Verification items for the finished model (mm, model axes). Face numbers are marked on the shaded views. A direction names the side the tool comes from. Round coordinates to 2 decimals unless told otherwise and drop trailing zeros. Write each loop counter-clockwise with the first axis right and the second up, starting at its lowest first coordinate (ties: lowest second). Pieces come first, ordered by that corner, then holes. Notation, with made-up numbers: M 2,58 L 31,58 A23 cw 31,87 Z; hole C 60.25,87 d3. An arc over 180 degrees is marked long. One line per item, written item: value. Start each with the question number.
Item 1: Gauge pin test, flat ends, axial feed: pin 1 (3.5 mm diameter, centred on x = 1, y = -17.5, fed in from +Z); pin 2 (2 mm diameter, centred on y = -5, z = 11, fed in from +X); pin 3 (1.6 mm diameter, centred on y = -19, z = -3.5, fed in from -X); pin 4 (13 mm diameter, centred on x = 19.64, z = -15, fed in from +Y). Record the tip position at first contact, or that the pin passes through.
Item 2: Tool access check on the marked faces 1 and 2. Record the directions out of +Z, -Z, +X, -X, +Y, -Y that give a thin tool (end or side, any length) a straight path to the whole face; none if there is none.
Item 3: Section check B-B, the plane y = -14. Record the cut outline in (x, z).
Item 4: Section check D-D, the plane x = 23. Record the cut outline in (y, z), then the cut area to 3 significant figures.
Item 5: Section check A-A, the plane x = 1. Record the cut outline in (y, z), then the cut area to 3 significant figures.
Item 6: Thickness scan on probe 1 along X at (y, z) = (-19, 15); probe 2 along X at (y, z) = (-1, 5.5); probe 3 along Y at (x, z) = (8.5, 0). Record the ranges inside material, lowest first. Write a range as from..to.
Item 7: Section check C-C, the plane z = 0. Record the cut outline in (x, y).
from build123d import *

# Parameters (mm, degrees)
SKETCH1_R           = 2.5
SKETCH1_W           = 35
SKETCH1_H           = 8
BOSS_EXTRUDE1_DEPTH = 1.5
BOSS_EXTRUDE2_DEPTH = 30
FILLET1_R           = 5
SKETCH2_R           = 5
SKETCH2_W           = 7
SKETCH2_H           = 35
CUT_EXTRUDE1_DEPTH  = 30


with BuildPart() as part:
    # Sketch1 → Boss-Extrude1 (new body)
    with BuildSketch(Plane(origin=(0, 0, 0), x_dir=(0, 0, -1), z_dir=(1, 0, 0))):
        with BuildLine():
            Line((25, 0), (15, 0))
            ThreePointArc((15, 0), (0, 15), (-15, 0))
            Line((-15, 0), (-25, 0))
            Line((-25, 0), (-25, -20))
            Line((-25, -20), (25, -20))
            Line((25, -20), (25, 0))
        make_face()
        Circle(SKETCH1_R, mode=Mode.SUBTRACT)
        with Locations((0, -14.5)):
            Rectangle(SKETCH1_W, SKETCH1_H, mode=Mode.SUBTRACT)
    extrude(amount=-BOSS_EXTRUDE1_DEPTH)

    # Sketch1_3 → Boss-Extrude2 (add)
    with BuildSketch(Plane(origin=(0, 0, 0), x_dir=(0, 0, -1), z_dir=(1, 0, 0))):
        Polygon((25, -20), (25, -18.5), (17.5, -18.5), (-17.5, -18.5), (-25, -18.5), (-25, -20), align=None)
    extrude(amount=BOSS_EXTRUDE2_DEPTH)

    # Fillet1
    fillet1_edges = [part.edges().sort_by_distance(p)[0] for p in [
        (-0.75, 0, -25),
        (-0.75, 0, 25),
        (-0.75, 0, 15),
        (-0.75, 0, -15),
    ]]
    fillet(fillet1_edges, radius=FILLET1_R)

    # Sketch2 → Cut-Extrude1 (cut)
    with BuildSketch(Plane(origin=(0, -18.5, 0), x_dir=(1, 0, 0), z_dir=(0, 1, 0))):
        with Locations(Location((19.642277283, 15, 0), (0, 0, 270))):
            Circle(SKETCH2_R)
        with Locations(Location((19.642277283, -15, 0), (0, 0, 270))):
            Circle(SKETCH2_R)
        with Locations((2, 0)):
            Rectangle(SKETCH2_W, SKETCH2_H)
    extrude(amount=-CUT_EXTRUDE1_DEPTH, mode=Mode.SUBTRACT)


solid = part.part
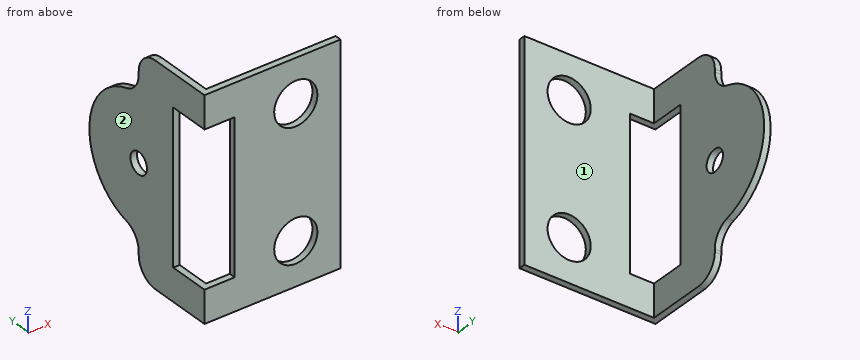
Response values:
1. pin 1: stops at z = 25
1. pin 2: stops at x = 0
1. pin 3: stops at x = 5.5
1. pin 4: stops at y = -18.5
2. face 1: +Z, -Z, +X, +Y
2. face 2: +Z, -Z, -X, +Y, -Y
3. outline: M -1.5,-25 L 0,-25 L 0,-17.5 L -1.5,-17.5 Z; M -1.5,17.5 L 0,17.5 L 0,25 L -1.5,25 Z
4. outline: M -20,-25 L -18.5,-25 L -18.5,-18.7 L -20,-18.7 Z; M -20,-11.3 L -18.5,-11.3 L -18.5,11.3 L -20,11.3 Z; M -20,18.7 L -18.5,18.7 L -18.5,25 L -20,25 Z
4. area: 52.8 mm2
5. outline: M -20,-25 L -18.5,-25 L -18.5,-17.5 L -20,-17.5 Z; M -20,17.5 L -18.5,17.5 L -18.5,25 L -20,25 Z
5. area: 22.5 mm2
6. probe 1: x = 5.5..14.64, 24.64..30
6. probe 2: x = -1.5..0
6. probe 3: y = -20..-18.5
7. outline: M -1.5,-10.5 L 0,-10.5 L 0,-2.5 L -1.5,-2.5 Z; M -1.5,2.5 L 0,2.5 L 0,15 L -1.5,15 Z; M 5.5,-20 L 30,-20 L 30,-18.5 L 5.5,-18.5 Z
